Model file for the job. Use its own axes, mm. Face numbers are marked on the shaded views. A direction names the side the tool comes from. Give positions to 0.01 mm unless a question says otherwise; leave off trailing zeros. Loops run counter-clockwise (first coordinate to the right, second up) from the corner with the lowest first, then second, coordinate; pieces in that order, holes last. Notation, with made-up numbers: M 67,75 L 72,75 A30 ccw 72,97 Z; hole C 7.25,88.5 d2. An arc over 180 degrees is marked long. Answer in a Markdown table with one row per item.
```python
from build123d import *

# Parameters (mm, degrees)
SKETCH1_W               = 80.4
SKETCH1_H               = 57
BOSS_EXTRUDE1_DEPTH     = 17
SKETCH2_R               = 3.1
BOSS_EXTRUDE2_DEPTH     = 17
SKETCH3_W               = 57
SKETCH3_H               = 18
BOSS_EXTRUDE3_DEPTH     = 10.8
CUT_EXTRUDE1_DEPTH      = 15
CUT_EXTRUDE2_DEPTH      = 60.868940194
CUT_EXTRUDE2_DEPTH_BACK = 60.868940194
SKETCH5_R               = 1.1


with BuildPart() as part:
    # Sketch1 → Boss-Extrude1 (new body)
    with BuildSketch(Plane(origin=(0, 0, 0), x_dir=(0, 1, 0), z_dir=(0, 0, 1))):
        Rectangle(SKETCH1_W, SKETCH1_H)
    extrude(amount=BOSS_EXTRUDE1_DEPTH)

    # Sketch2 → Boss-Extrude2 (add)
    with BuildSketch(Plane.XY.offset(17)):
        with Locations((-21.25, 32.95)):
            Circle(SKETCH2_R)
    extrude(amount=BOSS_EXTRUDE2_DEPTH)

    # Sketch3 → Boss-Extrude3 (add)
    with BuildSketch(Plane(origin=(0, 0, 0), x_dir=(1, 0, 0), z_dir=(0, 0, -1))):
        with Locations((0, 31.2)):
            Rectangle(SKETCH3_W, SKETCH3_H)
    extrude(amount=BOSS_EXTRUDE3_DEPTH)

    # Sketch4 → Cut-Extrude1 (cut)
    with BuildSketch(Plane.XY.offset(17)):
        Polygon((-14, 40.2), (-14, 25.7), (-28.5, 25.7), (-28.5, -40.2), (28.5, -40.2), (28.5, 40.2), align=None)
    extrude(amount=-CUT_EXTRUDE1_DEPTH, mode=Mode.SUBTRACT)

    # Sketch5 → Cut-Extrude2 (cut, two sides: drawn at the far end of the back side and taken through both)
    with BuildSketch(Plane(origin=(0, 0, 0), x_dir=(1, 0, 0), z_dir=(0, 0, -1)).offset(-CUT_EXTRUDE2_DEPTH_BACK)):
        with Locations((1.5, -35.6)):
            Circle(SKETCH5_R)
        with Locations((-10.5, 18.877250546)):
            Circle(SKETCH5_R)
        with Locations((12.249999272, 18.87149398)):
            Circle(SKETCH5_R)
    extrude(amount=CUT_EXTRUDE2_DEPTH + CUT_EXTRUDE2_DEPTH_BACK, mode=Mode.SUBTRACT)


solid = part.part
```
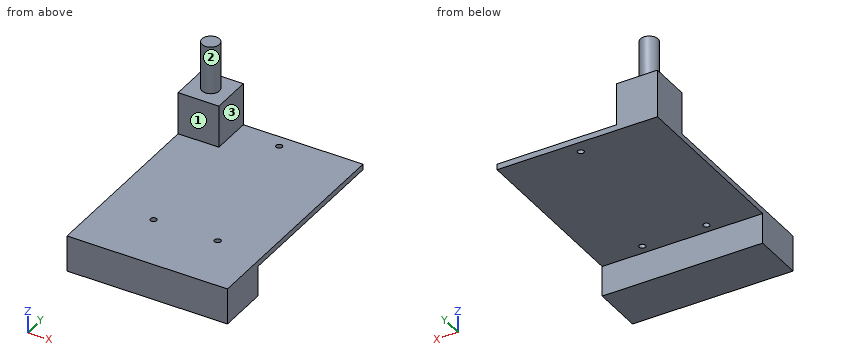
(1) Saw through at D-D, the plane z = 22. Give the cut face in (x, y).
Established:
| item | result |
|---|---|
| outline | C -21.25,32.95 d6.2 |
(2) Saw through at A-A, the plane x = 12.25. Give the cut face in (y, z).
Established:
| item | result |
|---|---|
| outline | M -40.2,-10.8 L -22.2,-10.8 L -22.2,0 L -19.97,0 L -19.97,2 L -40.2,2 Z; M -17.77,0 L 40.2,0 L 40.2,2 L -17.77,2 Z |
(3) Wall check: L1, parallel to Y at x = 1.5, z = 1.4; L2, parallel to Z at x = 17, y = 1; L3, parallel to Y at x = -24, z = 15. Give the ranges that are in metal, low to high.
Established:
| item | result |
|---|---|
| L1 | y = -40.2 to 34.5, 36.7 to 40.2 |
| L2 | z = 0 to 2 |
| L3 | y = 25.7 to 40.2 |
(4) Flat gauge pins, fed straight in: P1, Ø8, axis at x = -2, y = -11, coming from the -Z side; P2, Ø12, axis at y = -25.5, z = 9, coming from the -X side; P3, Ø7, axis at x = -25, z = 7.5, coming from the -Y side; P4, Ø1.5, axis at x = -21, y = 18, coming from the +Z side. Where does each tip first touch, or does it go through?
Established:
| item | result |
|---|---|
| P1 | stops at z = 0 |
| P2 | passes through |
| P3 | stops at y = 25.7 |
| P4 | stops at z = 2 |
(5) Saw through at C-C, the plane x = -20. Give the cut face in (y, z), and give its area (3 significant figures).
Established:
| item | result |
|---|---|
| outline | M -40.2,-10.8 L -22.2,-10.8 L -22.2,0 L 40.2,0 L 40.2,17 L 35.79,17 L 35.79,34 L 30.11,34 L 30.11,17 L 25.7,17 L 25.7,2 L -40.2,2 Z |
| area | 669 mm2 |
(6) Saw through at B-B, the plane y = 32.95. Give the cut face in (x, z).
Established:
| item | result |
|---|---|
| outline | M -28.5,0 L 28.5,0 L 28.5,2 L -14,2 L -14,17 L -18.15,17 L -18.15,34 L -24.35,34 L -24.35,17 L -28.5,17 Z |
(7) Which spindle directions (+Z, -Z, +X, -X, +Y, -Y) get a long thin tool onto all of the face, cutting with end or side? Do the marked faces 1, 2 and 3. Say none if no direction does.
Established:
| item | result |
|---|---|
| face 1 | +Z, +X, -X, -Y |
| face 2 | +Z |
| face 3 | +Z, +X, +Y, -Y |
